```python
from build123d import *

# Parameters (mm, degrees)
BOSS_EXTRU_2_DEPTH      = 6
ESQUISSE3_R             = 1.5
ENL_V_MAT_EXTRU_1_DEPTH = 48.391982444


with BuildPart() as part:
    # Esquisse1 → Boss.-Extru.2 (new body)
    with BuildSketch(Plane(origin=(0, 0, 0), x_dir=(1, 0, 0), z_dir=(0, 1, 0))):
        with BuildLine():
            Line((24, 0.5), (24, -10.5))
            Line((24, -10.5), (41, -10.5))
            ThreePointArc((41, -10.5), (40.121320344, -8.378679656), (38, -7.5))
            Line((38, -7.5), (28, -7.5))
            Line((28, -7.5), (28, 0.5))
            ThreePointArc((28, 0.5), (13, 15.5), (-2, 0.5))
            Line((-2, 0.5), (-2, -7.5))
            Line((-2, -7.5), (-12, -7.5))
            ThreePointArc((-12, -7.5), (-14.121320344, -8.378679656), (-15, -10.5))
            Line((-15, -10.5), (2, -10.5))
            Line((2, -10.5), (2, 0.5))
            ThreePointArc((2, 0.5), (13, 11.5), (24, 0.5))
        make_face()
    extrude(amount=BOSS_EXTRU_2_DEPTH)

    # Esquisse3 → Enlèv. mat.-Extru.1 (cut, through all)
    with BuildSketch(Plane(origin=(0, 0, 7.5), x_dir=(-1, 0, 0), z_dir=(0, 0, -1))):
        with Locations((-33, 3)):
            Circle(ESQUISSE3_R)
        with Locations(Location((7, 3, 0), (0, 0, 180))):
            Circle(ESQUISSE3_R)
    extrude(amount=-ENL_V_MAT_EXTRU_1_DEPTH, mode=Mode.SUBTRACT)


solid = part.part
```
Input: part model. Units: mm. Frame: model coordinates. A direction names the side the tool comes from. Round coordinates to 2 decimals unless told otherwise and drop trailing zeros. Loops run counter-clockwise (first coordinate to the right, second up) from the corner with the lowest first, then second, coordinate; pieces in that order, holes last. Notation, with made-up numbers: (-16, -32.75) -> (-2, -32.75) arc R17 cw to (-2, -8.75) -> close; hole circle Ø8 at (-22.5, 18.5). An arc over 180 degrees is marked (long way). Use one line per item in the form item = value. Start each with the question number.
Item 1: Contact query for flat-ended pins moving along their axis: pin 1 Ø5 at (x, z) = (16.5, -9.5) entering from +Y; pin 2 Ø1.8 at (y, z) = (2.5, 4.5) entering from +X; pin 3 Ø1.8 at (y, z) = (2, 7.5) entering from +X; pin 4 Ø3 at (x, y) = (-9, 4) entering from -Z. Output: stop coordinate, or through.
Item 2: Mould query, pull axis Y, two halves, no side actions, for faces 6 (the face through (34.2, 2.1, 9)), 7 (the face through (13.33, 2.958, -15.496)), 8 (the face through (2, 6, -4)), 9 (the face through (-8.11, 1.99, 8.98)). Classes: pulls with the +Y half, pulls with the -Y half, needs draft (parallel to the pull), parting line crosses it, or undercut.
Item 3: Material intervals for L1, parallel to Y at x = -7, z = 9.7; L2, parallel to X at y = 3.55, z = 0.5; L3, parallel to Z at x = -12, y = 3.35, sorted ascending. Write a range as from..to.
Item 4: Section query B-B on x = 33. Return the cut outline in (y, z).
Item 5: Section query D-D on y = 0.75. Return the cut outline in (x, z), then the cut area to 4 significant figures.
Item 6: Section query A-A on z = 2. Return the cut outline in (x, y).
Item 7: Set-up query: faces 1 (the face through (32, 1.6, 7.5)), 2 (the face through (2, 0, -4)), 3 (the face through (30, 3, 10.5)), 4 (the face through (2, 3, 5)), 5 (the face through (-2, 3, 3)). Return all of +Z, -Z, +X, -X, +Y, -Y with unobstructed straight access to the full face (end or side cutting, diameter ignored); none if empty.
Item 8: Section query C-C on y = 3.95. Return the cut outline in (x, z), then the cut area to 3 significant figures.
Ans:
q1.pin_1 = 6
q1.pin_2 = 28
q1.pin_3 = 40.14
q1.pin_4 = 7.5
q2.face_6 = undercut
q2.face_7 = needs draft
q2.face_8 = pulls with the +Y half
q2.face_9 = undercut
q3.L1 = 0..1.5, 4.5..6
q3.L2 = -2..2, 24..28
q3.L3 = 7.5..10.5
q4.outline = (0, 7.5) -> (1.5, 7.5) -> (1.5, 10.5) -> (0, 10.5) -> close; (4.5, 7.5) -> (6, 7.5) -> (6, 10.5) -> (4.5, 10.5) -> close
q5.outline = (-15, 10.5) arc R3 ccw to (-12, 7.5) -> (-2, 7.5) -> (-2, -0.5) arc R15 ccw to (28, -0.5) -> (28, 7.5) -> (38, 7.5) arc R3 ccw to (41, 10.5) -> (24, 10.5) -> (24, -0.5) arc R11 cw to (2, -0.5) -> (2, 10.5) -> close
q5.area = 325.5 mm^2
q6.outline = (-2, 0) -> (2, 0) -> (2, 6) -> (-2, 6) -> close; (24, 0) -> (28, 0) -> (28, 6) -> (24, 6) -> close
q7.face_1 = -Z, +X, +Y, -Y
q7.face_2 = +Z, -Z, +X, -X, -Y
q7.face_3 = +Z, +X, -X, +Y, -Y
q7.face_4 = +Z, +Y, -Y
q7.face_5 = -Z, -X, +Y, -Y
q8.outline = (-15, 10.5) arc R3 ccw to (-12, 7.5) -> (-8.16, 7.5) -> (-8.16, 10.5) -> close; (-5.84, 7.5) -> (-2, 7.5) -> (-2, -0.5) arc R15 ccw to (28, -0.5) -> (28, 7.5) -> (31.84, 7.5) -> (31.84, 10.5) -> (24, 10.5) -> (24, -0.5) arc R11 cw to (2, -0.5) -> (2, 10.5) -> (-5.84, 10.5) -> close; (34.16, 7.5) -> (38, 7.5) arc R3 ccw to (41, 10.5) -> (34.16, 10.5) -> close
q8.area = 312 mm^2
